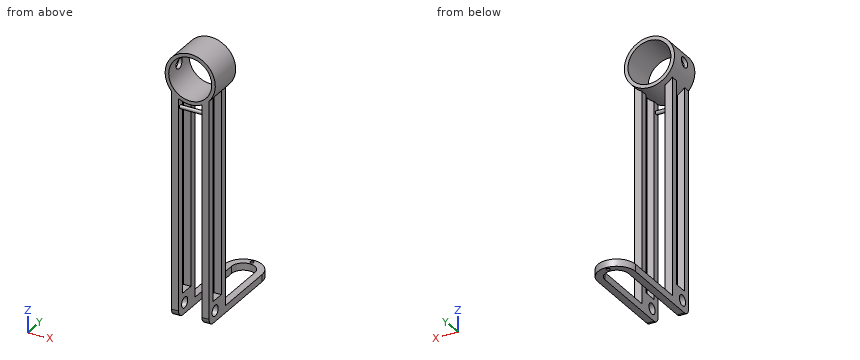
Autodesk Inventor part; units mm, degrees
ref_plane "Work Plane2" through (0, 0, 60) normal (0, 0, 1) x (1, 0, 0)
ref_plane "XZ Plane" through (0, 0, 0) normal (0, 1, 0) x (-1, 0, 0)
sketch "Sketch1" plane through (0, 0, 0) normal (0, 0, 1) x (1, 0, 0)
  line L0 (0, 0) -> (15, 0)
  line L1 (0, 0) -> (2.25, 0)
  line L2 (2.25, 0) -> (2.25, 4.6954)
  line L3 (2.25, 0) -> (4.25, 0)
  line L4 (4.25, 0) -> (4.25, 4.6954)
  line L5 (0, 0) -> (4.5, 0)
  line L6 (0, 0) -> (1.7131, 0)
  line L7 (0, 0) -> (2, 0)
  line L8 (2, 0) -> (2, -1.4268)
  line L9 (4.5, 0) -> (4.5, -1.5938)
  line L10 (0, 0) -> (10.5, 0)
  line L11 (10.5, 0) -> (10.5, -1.4268)
  line L12 (0, 0) -> (10.75, 0)
  line L13 (10.75, 0) -> (10.75, 3.2646)
  line L14 (10.75, 0) -> (12.75, 0)
  line L15 (12.75, 0) -> (12.75, 3.2646)
  line L16 (0, 0) -> (13, 0)
  line L17 (13, 0) -> (13, -1.4268)
  line L18 (12.75, 0) -> (12.75, 2)
  line L19 (12.75, 2) -> (10.75, 2)
  line L20 (10.75, 0) -> (12.75, 0)
  line L21 (4.25, 0) -> (4.25, 2)
  line L22 (4.25, 2) -> (2.25, 2)
  dimension "d0" = 15
  dimension "d1" = 2.25
  dimension "d2" = 2
  dimension "d3" = 4.5
  dimension "d4" = 2
  dimension "d5" = 10.5
  dimension "d6" = 10.75
  dimension "d7" = 2
  dimension "d8" = 13
  dimension "d9" = 2
  dimension "d10" = 2
extrude "Extrusion1" add sketch "Sketch1" along normal blind 60
sketch "Sketch2" plane through (2.25, 2, 0) normal (0, 1, 0) x (1, 0, 0)
  line L0 (2, 0) -> (0, 0)
  line L1 (0, 0) -> (0, -6)
  line L2 (0, -6) -> (2, -6)
  line L3 (2, -6) -> (2, 0)
  point P0 (-2.25, 0)
  dimension "d13" = 2
  dimension "d14" = 6
extrude "Extrusion2" add sketch "Sketch2" along normal blind 4
sketch "Sketch3" plane through (2.25, 0, 60) normal (-1, 0, 0) x (0, 0, 1)
  line L0 (-60, 0) -> (-60, 6)
  line L1 (-60, 0) -> (-60, 6)
  line L2 (-60, 6) -> (-54, 6)
  line L3 (-54, 2) -> (-54, 6)
  circle A0 centre (-57, 3) radius 1.5
  dimension "d17" = 6
  dimension "d18" = 3
extrude "Extrusion3" cut sketch "Sketch3" against normal blind 6
sketch "Sketch4" plane through (2.25, 6, 0) normal (0, 1, 0) x (1, 0, 0)
  line L0 (0, 0) -> (2, 0)
  line L1 (2, 0) -> (2, -2)
  line L2 (2, -2) -> (0, -2)
  line L3 (0, -2) -> (0, 0)
  point P0 (-2.25, 0)
  dimension "d22" = 2
  dimension "d23" = 2
extrude "Extrusion4" add sketch "Sketch4" along normal blind 20
sketch "Sketch5" plane through (10.75, 2, 0) normal (0, 1, 0) x (1, 0, 0)
  line L0 (0, 0) -> (0, -60)
  line L1 (2, 0) -> (0, 0)
  line L2 (0, 0) -> (0, -6)
  line L3 (0, -6) -> (2, -6)
  line L4 (2, -6) -> (2, 0)
  point P0 (-10.75, 0)
  dimension "d27" = 6
extrude "Extrusion5" add sketch "Sketch5" along normal blind 4
sketch "Sketch6" plane through (12.75, 0, 60) normal (1, 0, 0) x (0, 0, -1)
  line L0 (54, 6) -> (60, 0)
  circle A0 centre (57, 3) radius 1.5
  circle A1 centre (57, 3) radius 1.5
extrude "Extrusion6" cut sketch "Sketch6" against normal blind 4
sketch "Sketch7" plane through (10.75, 6, 0) normal (0, 1, 0) x (1, 0, 0)
  line L0 (0, 0) -> (2, 0)
  line L1 (2, 0) -> (2, -2)
  line L2 (2, -2) -> (0, -2)
  line L3 (0, -2) -> (0, 0)
  point P0 (-10.75, 0)
extrude "Extrusion7" add sketch "Sketch7" along normal blind 20
ref_plane "Work Plane1" through (0, 0, 0) normal (0, 0, 1) x (1, 0, 0)
sketch "Sketch8" plane through (0, 0, 0) normal (0, 0, 1) x (1, 0, 0)
  arc A0 (12.75, 26) -> (2.25, 26) centre (7.5, 26) ccw
  arc A1 (10.75, 26) -> (4.25, 26) centre (7.5, 26) ccw
  line L0 (12.75, 0) -> (12.75, 26)
  line L1 (12.75, 26) -> (10.75, 26)
  line L2 (4.25, 26) -> (2.25, 26)
  line L3 (4.25, 26) -> (2.25, 26)
  line L4 (12.75, 26) -> (10.75, 26)
  line L5 (4.25, 26) -> (2.25, 26)
  arc A2 (10.75, 26) -> (4.25, 26) centre (7.5, 26) ccw
  arc A3 (12.75, 26) -> (2.25, 26) centre (7.5, 26) ccw
  point P0 (0, 0)
  point P1 (12.75, 2)
extrude "Extrusion8" add sketch "Sketch8" along normal blind 2
ref_plane "Work Plane2" through (0, 0, 60) normal (0, 0, 1) x (1, 0, 0)
sketch "Sketch9" plane through (0, 0, 0) normal (0, 1, 0) x (-1, 0, 0)
  line L0 (-2.25, 60) -> (-12.75, 60)
  line L1 (-7.5, 60) -> (-0.5, 60) construction
  circle A0 centre (-7.5, 67) radius 6
  circle A1 centre (-7.5, 67) radius 7
  point P0 (0, 0)
extrude "Extrusion9" add sketch "Sketch9" along normal blind 10
sketch "Sketch10" plane through (0, 0, 60) normal (0, 0, 1) x (1, 0, 0)
  line L0 (2.25, 0) -> (4.25, 0)
  line L1 (4.25, 0) -> (4.25, 2)
  line L2 (4.25, 2) -> (2.25, 2)
  line L3 (2.25, 2) -> (2.25, 0)
  point P0 (0, 0)
extrude "Extrusion10" add sketch "Sketch10" along normal blind 1.5
sketch "Sketch11" plane through (0, 0, 61.5) normal (0, 0, 1) x (1, 0, 0)
  line L0 (2.25, 2) -> (3.1699, 2)
  line L1 (3.1699, 2) -> (3.1699, 0)
  line L2 (3.1699, 0) -> (2.25, 0)
  line L3 (2.25, 0) -> (3.1699, 0)
  line L4 (2.25, 0) -> (2.25, 2)
  point P0 (0, 0)
extrude "Extrusion11" add sketch "Sketch11" along normal blind 1
sketch "Sketch12" plane through (0, 0, 60) normal (0, 0, 1) x (1, 0, 0)
  line L0 (12.75, 0) -> (10.75, 0)
  line L1 (10.75, 0) -> (10.75, 2)
  line L2 (10.75, 2) -> (12.75, 2)
  line L3 (12.75, 2) -> (12.75, 0)
  point P0 (0, 0)
extrude "Extrusion12" add sketch "Sketch12" along normal blind 1.5
sketch "Sketch13" plane through (0, 0, 61.5) normal (0, 0, 1) x (1, 0, 0)
  line L0 (12.75, 0) -> (11.8301, 0)
  line L1 (11.8301, 0) -> (11.8301, 2)
  line L2 (11.8301, 2) -> (12.75, 2)
  line L3 (12.75, 2) -> (12.75, 0)
  point P0 (0, 0)
extrude "Extrusion13" add sketch "Sketch13" along normal blind 1
sketch "Sketch14" plane through (2.25, 6, 2) normal (0, 0, 1) x (1, 0, 0)
  line L0 (0, 0) -> (2, 0)
  line L1 (2, 0) -> (2, 2)
  line L2 (2, 2) -> (0, 2)
  line L3 (0, 2) -> (0, 0)
  line L4 (8.5, 0) -> (10.5, 0)
  line L5 (10.5, 0) -> (10.5, 2)
  line L6 (10.5, 2) -> (8.5, 2)
  line L7 (8.5, 2) -> (8.5, 0)
  point P0 (-2.25, -6)
  dimension "d52" = 2
  dimension "d53" = 2
  dimension "d54" = 2
  dimension "d55" = 2
extrude "Extrusion14" add sketch "Sketch14" along normal blind 59.5
sketch "Sketch15" plane through (2.25, 6, 61.5) normal (0, 0, 1) x (1, 0, 0)
  line L0 (10.5, 0) -> (9.5801, 0)
  line L1 (9.5801, 0) -> (9.5801, 2)
  line L2 (9.5801, 2) -> (10.5, 2)
  line L3 (10.5, 2) -> (10.5, 0)
  point P0 (-2.25, -6)
extrude "Extrusion15" add sketch "Sketch15" along normal blind 1
sketch "Sketch16" plane through (2.25, 6, 61.5) normal (0, 0, 1) x (1, 0, 0)
  line L0 (0, 0) -> (0.9199, 0)
  line L1 (0.9199, 0) -> (0.9199, 2)
  line L2 (0.9199, 2) -> (0, 2)
  line L3 (0, 2) -> (0, 0)
  point P0 (-2.25, -6)
extrude "Extrusion16" add sketch "Sketch16" along normal blind 1
fillet "Fillet4" radius 2 2 edges at (3.25, 0, 0) (11.75, 0, 0)
sketch "Sketch17" plane through (0, 0, 0) normal (0, 0, -1) x (-1, 0, 0)
  line L0 (-2.25, 26) -> (-12.75, 26)
  line L1 (-7.5, 26) -> (-7.5, 31.25)
  arc A0 (-2.25, 26) -> (-12.75, 26) centre (-7.5, 26) ccw
  circle A1 centre (-7.5, 30.2901) radius 0.5
  point P0 (0, 0)
  dimension "d63" = 1
extrude "Extrusion17" cut sketch "Sketch17" against normal blind 2 contours A1 L1 | L1 A1
sketch "Sketch18" plane through (10.75, 2, 6) normal (-1, 0, 0) x (0, 0, 1)
  circle A0 centre (52.1755, -1.1123) radius 0.5
  point P0 (-6, -2)
  dimension "d66" = 1
extrude "Extrusion18" add sketch "Sketch18" along normal blind 8
ref_plane "Work Plane3" through (0.5, 0, 0) normal (1, 0, 0) x (0, 1, 0)
sketch "Sketch19" plane through (0.5, 0, 0) normal (1, 0, 0) x (0, 1, 0)
  point P0 (0, 0)
sketch "Sketch20" plane through (0.5, 0, 0) normal (1, 0, 0) x (0, 1, 0)
  line L0 (0, 74) -> (0, 62.3699)
  line L1 (10, 73) -> (10, 61)
  circle A0 centre (5, 67.4828) radius 1.5
  point P0 (0, 0)
  dimension "d70" = 3
extrude "Extrusion19" cut sketch "Sketch20" along normal mid plane 10
properties part number "arm"
Source: CAD feature listing. Evaluate the final solid. Frame: model axes, mm. Round coordinates to 2 decimals unless told otherwise and drop trailing zeros. Write each loop counter-clockwise with the first axis right and the second up, starting at its lowest first coordinate (ties: lowest second). Pieces come first, ordered by that corner, then holes. Notation, with made-up numbers: (-21, -40) - (-4, -40) arc R27 cw to (-4, -5) - close; hole circle Ø4 at (5.25, 32.5). An arc over 180 degrees is marked (long way). Use CSV: the item, a comma, the result in double quotes. Start each with the question number.
(1) Cut plane C-C, the plane x = 11.5. Return loops of the section in (y, z), and give its area (3 significant figures).
(2) Material intervals for probe 1 along Y at (x, z) = (11, 54); probe 2 along Y at (x, z) = (11.6, 3); probe 3 along Z at (x, y) = (7.5, 5.75), sorted ascending. Write a range as [from, to].
(3) First-contact query: pin 1 Ø4 at (y, z) = (3, 3) entering from -X; pin 2 Ø3 at (x, z) = (10.5, 58) entering from -Y; pin 3 Ø8 at (x, z) = (12.5, 24.5) entering from +Y; pin 4 Ø5 at (x, y) = (8, 18) entering from +Z. Flat tips, straight axial feed; report the tip coordinate or a pass-through.
(4) Cut plane B-B, the plane z = 35. Return loops of the section in (x, y).
(5) Cut plane A-A, the plane y = 17. Return loops of the section in (x, z), and give its area (3 significant figures).
Geometry says:
1,outline,"(0, 2) arc R2 ccw to (2, 0) - (29.4, 0) - (29.4, 2) - (8, 2) - (8, 61.26) - (10, 61.26) - (10, 62.53) - (0, 62.53) - close; (0, 71.47) - (10, 71.47) - (10, 72.74) - (0, 72.74) - close; hole circle Ø3 at (3, 3); hole (2, 6) - (6, 6) - (6, 61.26) - (2, 61.26) - close"
1,area,"329 mm²"
2,probe 1,"[0, 2], [6, 8]"
2,probe 2,"[0, 1.5], [4.5, 8]"
2,probe 3,"[60, 61], [73, 74]"
3,pin 1,"x = 2.25"
3,pin 2,"y = 0"
3,pin 3,"y = 8"
3,pin 4,"through"
4,outline,"(2.25, 0) - (4.25, 0) - (4.25, 2) - (2.25, 2) - close; (2.25, 6) - (4.25, 6) - (4.25, 8) - (2.25, 8) - close; (10.75, 0) - (12.75, 0) - (12.75, 2) - (10.75, 2) - close; (10.75, 6) - (12.75, 6) - (12.75, 8) - (10.75, 8) - close"
5,outline,"(2.25, 0) - (4.25, 0) - (4.25, 2) - (2.25, 2) - close; (10.75, 0) - (12.75, 0) - (12.75, 2) - (10.75, 2) - close"
5,area,"8.00 mm²"
